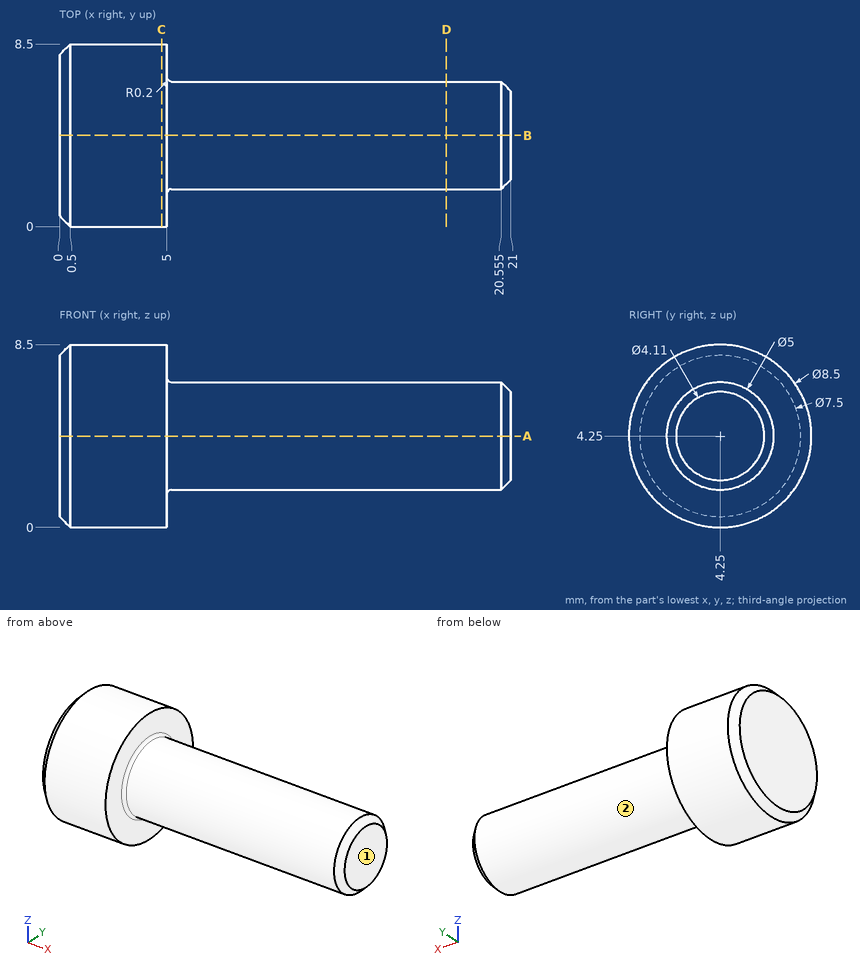
Study the drawing (mm; zero at the part's minimum x, y, z) and answer. A direction names the side the tool comes from. Coordinates: 2 decimals unless noted, no trailing zeros. Write each loop counter-clockwise with the first axis right and the second up, starting at its lowest first coordinate (ties: lowest second). Pieces come first, ordered by that corner, then holes. Notation, with made-up numbers: (42, 60.25) - (79, 60.25) arc R20 ccw to (79, 75.25) - close; hole circle Ø3 at (41, 35.25). An arc over 180 degrees is marked (long way). Answer as a JSON object with one key per item and string values.
Q1. Consider L1, parallel to X at y = 3, z = 7; L2, parallel to Y at x = 3.5, z = 2.25; L3, parallel to X at y = 5.75, z = 0.75. Determine where each line is inside the solid, lowest interval first. Write a range as from..to.
Results list:
{"L1": "x = 0..5", "L2": "y = 0.5..8", "L3": "x = 0.06..5"}
Q2. Which of the six approach directions +Z, -Z, +X, -X, +Y, -Y give full straight-line access (tool end or side, diameter ignored) to the marked faces 1 and 2?
Results list:
{"face 1": "+Z, -Z, +X, +Y, -Y", "face 2": "+X"}
Q3. Find section C-C (x = 4.75). Write down the section's boundary in (y, z).
Results list:
{"outline": "circle Ø8.5 at (4.25, 4.25)"}
Q4. Given pin 1 Ø3 at (x, y) = (2.5, 1) entering from +Z; pin 2 Ø3 at (x, y) = (5.5, 6.5) entering from -Z, each flat-ended and moving along its own axis, determine where each tip first touches the part or whether it passes through.
Results list:
{"pin 1": "stops at z = 8.12", "pin 2": "stops at z = 0.08"}
Q5. Find section D-D (x = 18). Write down the section's boundary in (y, z).
Results list:
{"outline": "circle Ø5 at (4.25, 4.25)"}
Q6. Find section A-A (z = 4.25). Write down the section's boundary in (x, y) (3 decimals).
Results list:
{"outline": "(0, 0.5) - (0.5, 0) - (5, 0) - (5, 1.55) arc R0.2 cw to (5.2, 1.75) - (20.555, 1.75) - (21, 2.195) - (21, 6.305) - (20.555, 6.75) - (5.2, 6.75) arc R0.2 cw to (5, 6.95) - (5, 8.5) - (0.5, 8.5) - (0, 8) - close"}
